Part model, mm, in its own coordinate system. A direction names the side the tool comes from. Round coordinates to 2 decimals unless told otherwise and drop trailing zeros. Write each loop counter-clockwise with the first axis right and the second up, starting at its lowest first coordinate (ties: lowest second). Pieces come first, ordered by that corner, then holes. Notation, with made-up numbers: (88.5, 46) -> (109.5, 46) arc R12 cw to (109.5, 59) -> close; hole circle Ø7 at (-20.75, -24.75). An arc over 180 degrees is marked (long way). Return JSON: item names as keys, results as strings. Group by question number.
```python
from build123d import *

# Parameters (mm, degrees)
SKETCH1_W           = 135
SKETCH1_H           = 210
BOSS_EXTRUDE1_DEPTH = 3
SKETCH2_R           = 3
SKETCH2_R_2         = 5
BOSS_EXTRUDE2_DEPTH = 3
SKETCH3_R           = 3
BOSS_EXTRUDE3_DEPTH = 3
SKETCH4_W           = 51.5
SKETCH4_H           = 121.5
BOSS_EXTRUDE4_DEPTH = 5
SKETCH5_W           = 48.3
SKETCH5_H           = 118.3
CUT_EXTRUDE1_DEPTH  = 2
FILLET1_R           = 2
FILLET2_R           = 3.6
FILLET3_R           = 5
SKETCH6_R           = 3.5
CUT_EXTRUDE2_DEPTH  = 5
SKETCH7_W           = 36
SKETCH7_H           = 6
BOSS_EXTRUDE5_DEPTH = 30
CUT_EXTRUDE3_REACH  = 228.481
CUT_EXTRUDE4_REACH  = 176.102
SKETCH9_R           = 1.625
SKETCH10_R          = 3.625
SKETCH10_R_2        = 3.75
SKETCH10_W          = 27
SKETCH10_H          = 60
CUT_EXTRUDE5_DEPTH  = 148.397421958
SKETCH11_W          = 5
SKETCH11_H          = 4
CUT_EXTRUDE6_DEPTH  = 148.397421958
SKETCH12_W          = 4
SKETCH12_H          = 4
BOSS_EXTRUDE6_DEPTH = 3
SKETCH13_W          = 10
SKETCH13_H          = 69
CUT_EXTRUDE7_DEPTH  = 151.113290551
SKETCH14_R          = 1.25
SKETCH14_R_2        = 1.625
CUT_EXTRUDE8_DEPTH  = 150.542636061
CUT_EXTRUDE9_REACH  = 189.206
CUT_EXTRUDE9_START  = -10
SKETCH15_W          = 6
SKETCH15_H          = 15
SKETCH16_R          = 1.8
CUT_EXTRUDE10_DEPTH = 151.113290551


with BuildPart() as part:
    # Sketch1 → Boss-Extrude1 (new body)
    with BuildSketch(Plane(origin=(0, 0, 0), x_dir=(1, 0, 0), z_dir=(0, 1, 0))):
        Rectangle(SKETCH1_W, SKETCH1_H)
    extrude(amount=BOSS_EXTRUDE1_DEPTH)

    # Sketch2 → Boss-Extrude2 (add)
    with BuildSketch(Plane(origin=(0, 3, 0), x_dir=(1, 0, 0), z_dir=(0, 1, 0))):
        with Locations(Location((-17, 95, 0), (0, 0, 90))):
            Circle(SKETCH2_R)
        with Locations(Location((17, 95, 0), (0, 0, 90))):
            Circle(SKETCH2_R)
        with Locations(Location((-17, 85, 0), (0, 0, 90))):
            Circle(SKETCH2_R)
        with Locations(Location((17, 85, 0), (0, 0, 90))):
            Circle(SKETCH2_R)
        with Locations(Location((-29, -35, 0), (0, 0, 90))):
            Circle(SKETCH2_R_2)
        with Locations(Location((29, -35, 0), (0, 0, 90))):
            Circle(SKETCH2_R_2)
        with Locations(Location((29, -84, 0), (0, 0, 90))):
            Circle(SKETCH2_R_2)
        with Locations(Location((-29, -84, 0), (0, 0, 90))):
            Circle(SKETCH2_R_2)
    extrude(amount=BOSS_EXTRUDE2_DEPTH)

    # Sketch3 → Boss-Extrude3 (add)
    with BuildSketch(Plane(origin=(0, 3, 0), x_dir=(1, 0, 0), z_dir=(0, 1, 0))):
        with Locations(Location((-64.5, -23, 0), (0, 0, 180))):
            Circle(SKETCH3_R)
        with Locations(Location((-38.5, -23, 0), (0, 0, 90))):
            Circle(SKETCH3_R)
        with Locations(Location((-38.5, -89, 0), (0, 0, 90))):
            Circle(SKETCH3_R)
        with Locations(Location((-64.5, -89, 0), (0, 0, 180))):
            Circle(SKETCH3_R)
    extrude(amount=BOSS_EXTRUDE3_DEPTH)

    # Sketch4 → Boss-Extrude4 (add)
    with BuildSketch(Plane.XZ):
        with Locations((73.25, 29.25)):
            Rectangle(SKETCH4_W, SKETCH4_H)
    extrude(amount=-BOSS_EXTRUDE4_DEPTH)

    # Sketch5 → Cut-Extrude1 (cut)
    with BuildSketch(Plane(origin=(0, 5, 0), x_dir=(1, 0, 0), z_dir=(0, 1, 0))):
        with Locations((73.25, -29.25)):
            Rectangle(SKETCH5_W, SKETCH5_H)
    extrude(amount=-CUT_EXTRUDE1_DEPTH, mode=Mode.SUBTRACT)

    # Fillet1
    fillet1_edges = [part.edges().sort_by_distance(p)[0] for p in [
        (49.1, 4, 88.4),
        (97.4, 4, 88.4),
        (97.4, 4, -29.9),
        (49.1, 4, -29.9),
    ]]
    fillet(fillet1_edges, radius=FILLET1_R)

    # Fillet2
    fillet2_edges = [part.edges().sort_by_distance(p)[0] for p in [
        (47.5, 4, -31.5),
        (47.5, 4, 90),
        (99, 2.5, -31.5),
        (99, 2.5, 90),
    ]]
    fillet(fillet2_edges, radius=FILLET2_R)

    # Fillet3
    fillet3_edges = [part.edges().sort_by_distance(p)[0] for p in [
        (67.5, 1.5, 90),
        (67.5, 1.5, 105),
        (-67.5, 1.5, 105),
        (-67.5, 1.5, -105),
        (67.5, 1.5, -105),
    ]]
    fillet(fillet3_edges, radius=FILLET3_R)

    # Sketch6 → Cut-Extrude2 (cut)
    with BuildSketch(Plane(origin=(0, 3, 0), x_dir=(1, 0, 0), z_dir=(0, 1, 0))):
        with Locations(Location((0, 45, 0), (0, 0, 270))):
            Circle(SKETCH6_R)
    extrude(amount=-CUT_EXTRUDE2_DEPTH, mode=Mode.SUBTRACT)

    # Sketch7 → Boss-Extrude5 (add)
    with BuildSketch(Plane(origin=(0, 3, 0), x_dir=(1, 0, 0), z_dir=(0, 1, 0))):
        with Locations((-46.494033915, 93.006908347)):
            Rectangle(SKETCH7_W, SKETCH7_H)
        with Locations((-46.494033915, 18.006908347)):
            Rectangle(SKETCH7_W, SKETCH7_H)
    extrude(amount=BOSS_EXTRUDE5_DEPTH)

    # Cut-Extrude3: up to this face of the body (flat: up to its plane)
    cut_extrude3_end = Plane(part.part.faces().sort_by_distance((-46.494033915, 18, -15.006908347))[0])
    # Sketch8 → Cut-Extrude3 (cut, up to the picked face)
    with BuildSketch(Plane(origin=(0, 0, -96.006908347), x_dir=(-1, 0, 0), z_dir=(0, 0, -1)), mode=Mode.PRIVATE) as cut_extrude3_sk1:
        Polygon((64.494033915, 33), (64.494033915, 6.129942315), (37.62397623, 33), align=None)
    cut_extrude3_tool1 = split(extrude(cut_extrude3_sk1.sketch, amount=-CUT_EXTRUDE3_REACH, mode=Mode.PRIVATE), bisect_by=cut_extrude3_end, keep=Keep.BOTH, mode=Mode.PRIVATE)
    add(cut_extrude3_tool1.solids().sort_by(Axis((-55.537348, 24.043314, -96.006908), (0, 0, 1)))[0], mode=Mode.SUBTRACT)

    # Cut-Extrude4: up to this plane
    cut_extrude4_end = Plane(origin=(-28.494033915, 33, -96.006908347), z_dir=(-1, 0, 0))
    # Sketch9 → Cut-Extrude4 (cut, up to the surface)
    with BuildSketch(Plane(origin=(-35.311988115, 35.311988115, 0), x_dir=(0, 0, 1), z_dir=(-0.7071067811865515, 0.7071067811865437, 0)), mode=Mode.PRIVATE) as cut_extrude4_sk1:
        with Locations(Location((-18.006908347, -5.269644948, 0), (0, 0, 270))):
            Circle(SKETCH9_R)
    cut_extrude4_tool1 = split(extrude(cut_extrude4_sk1.sketch, amount=-CUT_EXTRUDE4_REACH, mode=Mode.PRIVATE), bisect_by=cut_extrude4_end, keep=Keep.BOTH, mode=Mode.PRIVATE)
    add(cut_extrude4_tool1.solids().sort_by_distance((-39.03819, 31.585786, -18.006908))[0], mode=Mode.SUBTRACT)
    # Sketch9 → Cut-Extrude4 (cut, up to the surface)
    with BuildSketch(Plane(origin=(-35.311988115, 35.311988115, 0), x_dir=(0, 0, 1), z_dir=(-0.7071067811865515, 0.7071067811865437, 0)), mode=Mode.PRIVATE) as cut_extrude4_sk2:
        with Locations(Location((-93.006908347, -5.269644948, 0), (0, 0, 270))):
            Circle(SKETCH9_R)
    cut_extrude4_tool2 = split(extrude(cut_extrude4_sk2.sketch, amount=-CUT_EXTRUDE4_REACH, mode=Mode.PRIVATE), bisect_by=cut_extrude4_end, keep=Keep.BOTH, mode=Mode.PRIVATE)
    add(cut_extrude4_tool2.solids().sort_by_distance((-39.03819, 31.585786, -93.006908))[0], mode=Mode.SUBTRACT)

    # Sketch10 → Cut-Extrude5 (cut, through all)
    with BuildSketch(Plane(origin=(0, 3, 0), x_dir=(1, 0, 0), z_dir=(0, 1, 0))):
        with Locations(Location((-42.5, 0.006908347, 0), (0, 0, 270))):
            Circle(SKETCH10_R)
        with Locations(Location((-57.5, 0.006908347, 0), (0, 0, 270))):
            Circle(SKETCH10_R_2)
        with Locations((-51.5, -56)):
            Rectangle(SKETCH10_W, SKETCH10_H)
    extrude(amount=-CUT_EXTRUDE5_DEPTH, mode=Mode.SUBTRACT)

    # Sketch11 → Cut-Extrude6 (cut, through all)
    with BuildSketch(Plane(origin=(0, 3, 0), x_dir=(1, 0, 0), z_dir=(0, 1, 0))):
        with Locations((43, -25.75)):
            Rectangle(SKETCH11_W, SKETCH11_H)
        with Locations((43, -32.75)):
            Rectangle(SKETCH11_W, SKETCH11_H)
    extrude(amount=-CUT_EXTRUDE6_DEPTH, mode=Mode.SUBTRACT)

    # Sketch12 → Boss-Extrude6 (add)
    with BuildSketch(Plane.XZ):
        with Locations((101, 29.25)):
            Rectangle(SKETCH12_W, SKETCH12_H)
    extrude(amount=-BOSS_EXTRUDE6_DEPTH)

    # Sketch13 → Cut-Extrude7 (cut, through all)
    with BuildSketch(Plane(origin=(0, 3, 0), x_dir=(1, 0, 0), z_dir=(0, 1, 0))):
        with Locations((-30.494033915, 55.506908347)):
            Rectangle(SKETCH13_W, SKETCH13_H)
    extrude(amount=-CUT_EXTRUDE7_DEPTH, mode=Mode.SUBTRACT)

    # Sketch14 → Cut-Extrude8 (cut, through all)
    with BuildSketch(Plane(origin=(0, 6, 0), x_dir=(1, 0, 0), z_dir=(0, 1, 0))):
        with Locations(Location((-38.5, -89, 0), (0, 0, 270))):
            Circle(SKETCH14_R)
        with Locations(Location((-64.5, -89, 0), (0, 0, 270))):
            Circle(SKETCH14_R)
        with Locations(Location((-38.5, -23, 0), (0, 0, 270))):
            Circle(SKETCH14_R)
        with Locations(Location((-64.5, -23, 0), (0, 0, 270))):
            Circle(SKETCH14_R)
        with Locations(Location((-29, -35, 0), (0, 0, 270))):
            Circle(SKETCH14_R_2)
        with Locations(Location((-29, -84, 0), (0, 0, 270))):
            Circle(SKETCH14_R_2)
        with Locations(Location((29, -84, 0), (0, 0, 270))):
            Circle(SKETCH14_R_2)
        with Locations(Location((29, -35, 0), (0, 0, 270))):
            Circle(SKETCH14_R_2)
        with Locations(Location((17, 95, 0), (0, 0, 270))):
            Circle(SKETCH14_R_2)
        with Locations(Location((17, 85, 0), (0, 0, 270))):
            Circle(SKETCH14_R_2)
        with Locations(Location((-17, 85, 0), (0, 0, 270))):
            Circle(SKETCH14_R_2)
        with Locations(Location((-17, 95, 0), (0, 0, 270))):
            Circle(SKETCH14_R_2)
    extrude(amount=-CUT_EXTRUDE8_DEPTH, mode=Mode.SUBTRACT)

    # Cut-Extrude9: up to this face of the body (flat: up to its plane)
    cut_extrude9_end = Plane(part.part.faces().sort_by_distance((-28.494033915, 17.787931336, -93.006908347))[0])
    # Sketch15 → Cut-Extrude9 (cut, up to the picked face)
    with BuildSketch(Plane(origin=(-35.311988115, 35.311988115, 0), x_dir=(0, 0, 1), z_dir=(-0.7071067811865515, 0.7071067811865437, 0)).offset(CUT_EXTRUDE9_START), mode=Mode.PRIVATE) as cut_extrude9_sk1:
        with Locations((-93.006908347, -4.313800825)):
            Rectangle(SKETCH15_W, SKETCH15_H)
    cut_extrude9_tool1 = split(extrude(cut_extrude9_sk1.sketch, amount=-CUT_EXTRUDE9_REACH, mode=Mode.PRIVATE), bisect_by=cut_extrude9_end, keep=Keep.BOTH, mode=Mode.PRIVATE)
    # Sketch15 → Cut-Extrude9 (cut, up to the picked face)
    with BuildSketch(Plane(origin=(-35.311988115, 35.311988115, 0), x_dir=(0, 0, 1), z_dir=(-0.7071067811865515, 0.7071067811865437, 0)).offset(CUT_EXTRUDE9_START), mode=Mode.PRIVATE) as cut_extrude9_sk2:
        with Locations((-18.006908347, -4.313800825)):
            Rectangle(SKETCH15_W, SKETCH15_H)
    cut_extrude9_tool2 = split(extrude(cut_extrude9_sk2.sketch, amount=-CUT_EXTRUDE9_REACH, mode=Mode.PRIVATE), bisect_by=cut_extrude9_end, keep=Keep.BOTH, mode=Mode.PRIVATE)
    add(cut_extrude9_tool1.solids().sort_by(Axis((-31.291238, 25.190602, -93.006908), (0.7071067811865515, -0.7071067811865437, 0)))[0], mode=Mode.SUBTRACT)
    add(cut_extrude9_tool2.solids().sort_by(Axis((-31.291238, 25.190602, -18.006908), (0.7071067811865515, -0.7071067811865437, 0)))[0], mode=Mode.SUBTRACT)

    # Sketch16 → Cut-Extrude10 (cut, through all)
    with BuildSketch(Plane(origin=(0, 3, 0), x_dir=(1, 0, 0), z_dir=(0, 1, 0))):
        with Locations(Location((20, 0, 0), (0, 0, 270))):
            Circle(SKETCH16_R)
        with Locations(Location((-20, 0, 0), (0, 0, 270))):
            Circle(SKETCH16_R)
    extrude(amount=-CUT_EXTRUDE10_DEPTH, mode=Mode.SUBTRACT)


solid = part.part
```
Item 1: Two-plate mould, pull along X, no slides. Class faces 1 (the face through (-63.85, 4.48, 86.07)), 2 (the face through (-15.7, 6, -96.3)), 3 (the face through (66.07, 1.52, 103.5)): released by +X, released by -X, zero draft, split by the parting line, or undercut.
Item 2: Cut at B-B (z = 16.5). Write the cut outline in (x, y), then the cut area to 3 significant figures.
Item 3: Cut at A-A (z = 55.5). Write the cut outline in (x, y).
Item 4: Wall check: L1, parallel to X at y = 1.5, z = 0 (3 decimals); L2, parallel to X at y = 3.5, z = -95 (3 decimals); L3, parallel to X at y = 2.5, z = 76. Give the ranges that are in metal, low to high.
Item 5: Which spindle directions (+Z, -Z, +X, -X, +Y, -Y) get a long thin tool onto all of the face, cutting with end or side? Do faces 4 (the face through (-28.494, 30, -93)), 5 (the face through (-33.39, 23.09, -18.05)), 6 (the face through (-40.53, 4.48, 25.21)), 7 (the face through (-28.494, 7, -93)). Say none if no direction does.
Item 6: Cut at C-C (x = 6.5). Write the cut outline in (y, z).
Item 7: Flat gauge pins, fed straight in: P1, Ø8, axis at x = -31.5, z = 85, coming from the +Y side; P2, Ø1.5, axis at x = 20, y = 7.5, coming from the +Z side; P3, Ø1.5, axis at x = 73, y = 2, coming from the -Z side; P4, Ø1.6, axis at y = 4.5, z = 53, coming from the -X side. Where does each tip first touch, or does it go through?
Item 8: Cut at D-D (z = -73.5). Write the cut outline in (x, y).
Checks:
{
 "1": {"face 1": "undercut", "face 2": "zero draft", "face 3": "released by +X"},
 "2": {"outline": "(-67.5, 0) -> (99, 0) -> (99, 5) -> (97.4, 5) -> (97.4, 3) -> (49.1, 3) -> (49.1, 5) -> (47.5, 5) -> (47.5, 3) -> (-67.5, 3) -> close", "area": "506 mm2"},
 "3": {"outline": "(-67.5, 0) -> (-65, 0) -> (-65, 3) -> (-67.5, 3) -> close; (-38, 0) -> (99, 0) -> (99, 5) -> (97.4, 5) -> (97.4, 3) -> (49.1, 3) -> (49.1, 5) -> (47.5, 5) -> (47.5, 3) -> (-38, 3) -> close"},
 "4": {"L1": "x = -67.5 to -61.25, -53.75 to -46.125, -38.875 to -21.8, -18.2 to 18.2, 21.8 to 99", "L2": "x = -64.494 to -28.494, -20 to -18.625, -15.375 to -14, 14 to 15.375, 18.625 to 20", "L3": "x = -67.5 to -65, -38 to 99"},
 "5": {"face 4": "+Z, -Z, +X, +Y", "face 5": "+Z, -Z, +X", "face 6": "+Y", "face 7": "-Z, +Y"},
 "6": {"outline": "(0, -105) -> (3, -105) -> (3, 105) -> (0, 105) -> close"},
 "7": {"P1": "stops at y = 6", "P2": "passes through", "P3": "stops at z = -31.5", "P4": "stops at x = 47.5"},
 "8": {"outline": "(-67.5, 0) -> (-35.49, 0) -> (-35.49, 3) -> (-67.5, 3) -> close; (-25.49, 0) -> (67.5, 0) -> (67.5, 3) -> (-25.49, 3) -> close"}
}
